Autodesk Inventor part; units mm, degrees
ref_plane "MSC_PF1" through (0, 0, 0) normal (1, 0, 0) x (0, 1, 0)
ref_plane "MSC_PT1" through (0, 0, 0) normal (0, 0, -1) x (-1, 0, 0)
ref_plane "YZ Plane" through (0, 0, 0) normal (1, 0, 0) x (0, 1, 0)
sketch "Esquisse1" plane through (0, 0, 0) normal (0, 1, 0) x (-1, 0, 0)
  point P0 (0, 0)
sketch "Esquisse2" plane through (0, 0, 0) normal (0, 0, 1) x (1, 0, 0)
  point P0 (0, 0)
sketch "Esquisse3" plane through (0, 0, 0) normal (0, 0, 1) x (1, 0, 0)
  point P0 (0, 0)
sketch "Esquisse4" plane through (0, 0, 0) normal (0, 1, 0) x (-1, 0, 0)
  line L0 (-2.35, 0) -> (0, 0)
  line L1 (-2.35, -0.4) -> (-2.35, 0)
  line L2 (-1.25, -1.5) -> (-2.35, -0.4)
  line L3 (-1.25, -1.725) -> (-1.25, -1.5)
  line L4 (-1.025, -1.95) -> (-1.25, -1.725)
  line L5 (-1.25, -2.175) -> (-1.025, -1.95)
  line L6 (-1.25, -12) -> (-1.25, -2.175)
  line L7 (0, 0) -> (0, -12)
  line L8 (0, 3.3392) -> (0, -10.7) construction
  line L9 (0, 3.3392) -> (0, -10.7)
  line L10 (0, -15.0678) -> (0, 6.4071)
  line L11 (-1.25, -12) -> (0, -12)
  line L12 (0.47, 0) -> (-2.82, 0)
  dimension "d3" = 2.35
  dimension "d5" = 0.225
  dimension "d7" = 0.225
  dimension "d9" = 0.225
  dimension "d11" = 1.5
  dimension "d13" = 135
  dimension "d17" = 1.025
  dimension "d19" = 0
  dimension "d51" = 1.25
  dimension "d52" = 12
revolve "Révolution1" add sketch "Esquisse4" angle 360 about axis through (0, 0, 3.3392) along (0, 0, -1)
sketch "Esquisse5" plane through (0, 0, 0) normal (0, 1, 0) x (-1, 0, 0)
  line L0 (-1.45, 0) -> (0, 0)
  line L1 (-0.2417, -1.3636) -> (-1.45, 0)
  line L2 (0, -1.3636) -> (-0.2417, -1.3636)
  line L3 (0, 0) -> (0, -1.3636)
  line L4 (-1.25, -1.5) -> (1.25, -1.5) construction
  line L5 (-2.35, 0) -> (2.35, 0)
  line L6 (0, -1.8) -> (0, 0.3)
  dimension "d22" = 1.45
  dimension "d24" = 0.2417
  dimension "d26" = 1.3636
extrude "Extrusion1" cut sketch "Esquisse5" along normal mid plane 0.4833
pattern_circular "RéseauPolaire1" count 4 over 360 about axis through (0, 0, 0) along (0, 0, 1) of "Extrusion1"
sketch "Esquisse7" plane through (0, 0, 0) normal (0, 1, 0) x (-1, 0, 0)
  line L0 (0, -0.75) -> (-1.8125, 0)
  line L1 (0, 0) -> (0, -0.75)
  line L2 (-1.8125, 0) -> (0, 0)
  line L3 (-1.25, -1.5) -> (1.25, -1.5) construction
  line L4 (0, -1.8) -> (0, 0.3)
  line L5 (-2.35, 0) -> (2.35, 0)
  dimension "d33" = 1.8125
  dimension "d35" = 0.75
extrude "Extrusion2" cut sketch "Esquisse7" along normal mid plane 0.4833
pattern_circular "RéseauPolaire2" count 4 over 360 about axis through (0, 0, 0) along (0, 0, 1) of "Extrusion2"
fillet "Congé1" radius 0.45 1 edges at (-1.25, 0, -1.5)
thread "Filetage1"
ref_plane "MSC_PF1" through (0, 0, 0) normal (1, 0, 0) x (0, 1, 0)
ref_plane "MSC_PT1" through (0, 0, 0) normal (0, 0, -1) x (-1, 0, 0)
equation "\"d3\" = 0.5 * Dh"
equation "\"d5\" = msp_x"
equation "\"d7\" = ParA"
equation "\"d9\" = msp_x"
equation "\"d11\" = ParK"
equation "\"d17\" = 0.5 * msp_mdtds"
equation "\"d51\" = 0.5 * NND"
equation "\"d52\" = NLG"
equation "\"d22\" = 0.5 * M"
equation "\"d24\" = 0.0833333 * M"
equation "\"d26\" = 0.909091 * ParK"
equation "\"d27\" = 0.166667 * M"
equation "\"d33\" = 0.625 * M"
equation "\"d35\" = 0.5 * ParK"
equation "\"d36\" = 0.166667 * M"
equation "\"d41\" = 2 * msp_x"
equation "\"PTC\" = 0.45"
equation "\"NLG\" = 12"
equation "\"ParK\" = 1.5"
equation "\"NND\" = 2.5"
equation "\"M\" = 2.9"
equation "\"msp_mdtds\" = NND - PTC"
equation "\"Dh\" = 4.7"
equation "\"msp_x\" = 0.5 * PTC"
equation "\"ParA\" = 0.5 * PTC"
equation "\"r\" = 0.6"
equation "\"THREADDIA\" = NND"
equation "\"TEMPLATE\" = 1.2345"
properties part number "NF EN ISO 7046-2 H - M2.5x12 - 8.8 - H1" material "Acier inoxydable 440C"
Can you work these out from the model? Positions are in its coordinate system, mm. A direction names the side the tool comes from. Round coordinates to 2 decimals unless told otherwise and drop trailing zeros. Loops run counter-clockwise (first coordinate to the right, second up) from the corner with the lowest first, then second, coordinate; pieces in that order, holes last. Notation, with made-up numbers: (60.5, 31) - (110.5, 31) arc R24 cw to (110.5, 65) - close; hole circle Ø8 at (5, 83.25). An arc over 180 degrees is marked (long way). Answer in a Markdown table with one row per item. Add a question column.
Q1. Which directions (+Z, -Z, +X, -X, +Y, -Y) give clear straight access to the entire face, cutting with the end or side of a thin tool? Please do faces 1 (the cylindrical face through (-0.27, -1.22, -7.02)), 2 (the flat face through (0, 0, -12)), 3 (the flat face through (0.7, -0.242, -0.4)).
Q2. I want a section at B-B on z = -7.25. List the corners of the cut face in (x, y) for me.
Q3. I need wall thicknesses on L1, parallel to Z at x = 0, y = 0.1; L2, parallel to Y at x = 0, z = -8; L3, parallel to X at y = 0.05, z = -0.75. Which ranges of each line are inside material? Lowest first, please.
Q4. I want a section at A-A on z = -0.75. List the corners of the cut face in (x, y) for me.
Q5. For pin 1 Ø1 at (y, z) = (-1.5, -6.5) entering from +X; pin 2 Ø1.5 at (y, z) = (1, -0.5) entering from -X; pin 3 Ø2 at (y, z) = (-1, -3.5) entering from +X, each with a flat end and sliding along its axis, tell me the tip position at first contact or that it passes through.
A:
| question | item | result |
|---|---|---|
| 1 | face 1 | -Z |
| 1 | face 2 | -Z, +X, -X, +Y, -Y |
| 1 | face 3 | +Z |
| 2 | outline | circle Ø2.5 at (0, 0) |
| 3 | L1 | -12 to -1.36 |
| 3 | L2 | -1.25 to 1.25 |
| 3 | L3 | -2 to -0.79, 0.79 to 2 |
| 4 | outline | circle Ø4 at (0, 0); hole (-0.79, -0.24) - (-0.24, -0.24) - (-0.24, -0.79) - (0.24, -0.79) - (0.24, -0.24) - (0.79, -0.24) - (0.79, 0.24) - (0.24, 0.24) - (0.24, 0.79) - (-0.24, 0.79) - (-0.24, 0.24) - (-0.79, 0.24) - close |
| 5 | pin 1 | x = 0.75 |
| 5 | pin 2 | x = -2.34 |
| 5 | pin 3 | x = 1.25 |
